```python
from build123d import *

# Parameters (mm, degrees)
PAD_DEPTH       = 15
SKETCH001_R     = 2.75
POCKET_DEPTH    = 1.5
SKETCH002_R     = 2.75
POCKET001_DEPTH = 1.501


with BuildPart() as part:
    # Sketch → Pad (new body)
    with BuildSketch(Plane.XY):
        Polygon((-1.5, 1.5), (-23, 1.5), (-23, 0), (0, 0), (0, 23), (-1.5, 23), align=None)
    extrude(amount=PAD_DEPTH)

    # Sketch001 → Pocket (cut)
    with BuildSketch(Plane(origin=(0, 1.5, 0), x_dir=(-1, 0, 0), z_dir=(0, 1, 0))):
        with Locations((15.25, 7.5)):
            Circle(SKETCH001_R)
    extrude(amount=-POCKET_DEPTH, mode=Mode.SUBTRACT)

    # Sketch002 → Pocket001 (cut, through all)
    with BuildSketch(Plane(origin=(-1.5, 0, 0), x_dir=(0, -1, 0), z_dir=(-1, 0, 0))):
        with Locations((-15.25, 7.5)):
            Circle(SKETCH002_R)
    extrude(amount=-POCKET001_DEPTH, mode=Mode.SUBTRACT)


solid = part.part
```
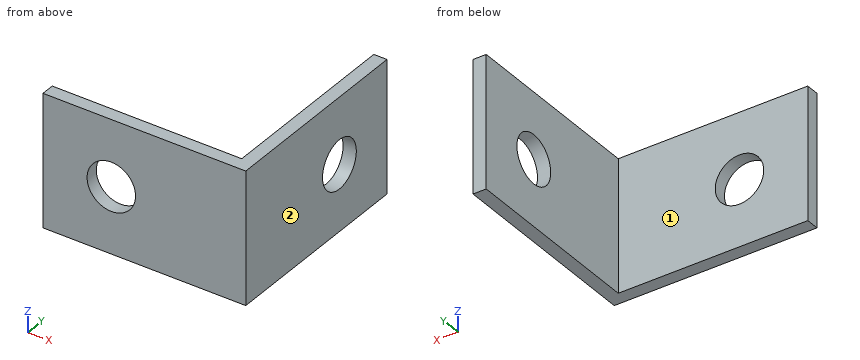
Check sheet for the modelled part. Datum: model origin and axes. Units: mm. Face numbers are marked on the shaded views. A direction names the side the tool comes from. Round coordinates to 2 decimals unless told otherwise and drop trailing zeros. Loops run counter-clockwise (first coordinate to the right, second up) from the corner with the lowest first, then second, coordinate; pieces in that order, holes last. Notation, with made-up numbers: (82.5, 16) -> (109.5, 16) arc R24 ccw to (109.5, 27) -> close; hole circle Ø9 at (-16, 9). An arc over 180 degrees is marked (long way). Write item = value, one per line. Start each with the question number.
1) Sectioned sample at A-A, the plane z = 7.5. Record the cut outline in (x, y).
2) Gauge pin test, flat ends, axial feed: pin 1 Ø4.5 at (y, z) = (7.5, 4.5) entering from -X; pin 2 Ø3 at (x, z) = (-12, 10.5) entering from +Y. Record the tip position at first contact, or that the pin passes through.
3) Set-up check for the marked faces 1 and 2: record each of +Z, -Z, +X, -X, +Y, -Y from which the full face is reachable in a straight line by a thin tool's end or side.
4) Sectioned sample at C-C, the plane y = 15.25. Record the cut outline in (x, z), plus the area to 4 significant figures.
5) Sectioned sample at D-D, the plane z = 3.5. Record the cut outline in (x, y).
6) Thickness scan on probe 1 along Z at (x, y) = (-15.25, 0.85); probe 2 along X at (y, z) = (19.5, 10.25); probe 3 along Y at (x, z) = (-8, 10.5). Record the ranges inside material, lowest first.
7) Sectioned sample at B-B, the plane x = -15.25. Record the cut outline in (y, z), plus the area to 4 significant figures.
Results are:
q1.outline = (-23, 0) -> (-18, 0) -> (-18, 1.5) -> (-23, 1.5) -> close; (-12.5, 0) -> (0, 0) -> (0, 12.5) -> (-1.5, 12.5) -> (-1.5, 1.5) -> (-12.5, 1.5) -> close; (-1.5, 18) -> (0, 18) -> (0, 23) -> (-1.5, 23) -> close
q2.pin_1 = -1.5
q2.pin_2 = 1.5
q3.face_1 = +Z, -Z, -X, +Y
q3.face_2 = +Z, -Z, +X, +Y, -Y
q4.outline = (-1.5, 0) -> (0, 0) -> (0, 4.75) -> (-1.5, 4.75) -> close; (-1.5, 10.25) -> (0, 10.25) -> (0, 15) -> (-1.5, 15) -> close
q4.area = 14.25 mm^2
q5.outline = (-23, 0) -> (0, 0) -> (0, 23) -> (-1.5, 23) -> (-1.5, 1.5) -> (-23, 1.5) -> close
q6.probe_1 = 0 to 4.75, 10.25 to 15
q6.probe_2 = -1.5 to 0
q6.probe_3 = 0 to 1.5
q7.outline = (0, 0) -> (1.5, 0) -> (1.5, 4.75) -> (0, 4.75) -> close; (0, 10.25) -> (1.5, 10.25) -> (1.5, 15) -> (0, 15) -> close
q7.area = 14.25 mm^2
